Model file for the job. Use its own axes, mm. A direction names the side the tool comes from. Coordinates: 2 decimals unless noted, no trailing zeros. Order: outer loops, then holes, each group sorted by start corner. A loop starts at its lowest first (then second) coordinate and runs counter-clockwise, first axis right, second up. Notation, with made-up numbers: (-13, 10.5) -> (-4, 10.5) arc R32 ccw to (-4, 40.5) -> close; hole circle Ø10 at (55.5, -20). An arc over 180 degrees is marked (long way). Use CSV: the item, a comma, the result in double quotes. Start each with the question number.
(1) Cut at B-B on x = 20. Write the cut outline in (y, z), plus the area to 3 significant figures.
(2) Tool access for faces 4 (the flat face through (33, 19.05, -60)), 5 (the cylindrical face through (31.91, 9.392, -74.446)), 6 (the flat face through (33, 19.05, 59)): list every direction of +Z, -Z, +X, -X, +Y, -Y with a clear straight run to the whole face (end or side of a thin tool).
(3) Probe L1, parallel to Z at x = 38, y = 7; L2, parallel to Y at x = 50, z = -64.5; L3, parallel to Z at x = 21.5, y = 41. List the from-to ranges inside material, lowest first.
(4) Cut at A-A on x = 41. Write the cut outline in (y, z).
(5) Cut at C-C on y = 14.5. Give the number of separate pieces and of enclosed holes in the cut face, plus the area to 3 significant figures.
(6) Pull direction Z, two halves, no side cores. Call faces 1 (the cylindrical face through (48.74, 59.68, -1.02)), 2 (the cylindrical face through (31.715, 9.392, 74.433)), 3 (the cylindrical face through (42.34, 9.39, 52.64)): pulls with the +Z half, pulls with the -Z half, needs draft (parallel to the pull), parting line crosses it, or undercut.
(7) Pin check, flat tips, straight feed: pin 1 Ø1.3 at (x, y) = (42, 1.5) entering from -Z; pin 2 Ø24 at (x, z) = (29, -59) entering from +Y; pin 3 Ø12 at (x, y) = (36.5, 43) entering from +Z. Stop position of each tip, or through.
(8) Cut at D-D on z = 0. Write the cut outline in (x, y), plus the area to 3 significant figures.
```python
from build123d import *

# Parameters (mm, degrees)
SKETCH1_R               = 4.7625
SKETCH1_R_2             = 4.445
BOSS_EXTRUDE1_DEPTH     = 76.2
CUT_EXTRUDE6_DEPTH      = 61.487180317
CUT_EXTRUDE7_DEPTH      = 7.187819683
CUT_EXTRUDE7_DEPTH_BACK = 61.487180417
SKETCH10_R              = 9.525
CUT_EXTRUDE8_DEPTH      = 41.6400001


with BuildPart() as part:
    # Sketch1 → Boss-Extrude1 (new body)
    with BuildSketch(Plane(origin=(0, 0, 0), x_dir=(1, 0, 0), z_dir=(0, 1, 0))):
        with BuildLine():
            ThreePointArc((38.550556967, -72.995596152), (82.55, 0), (38.550556967, 72.995596152))
            ThreePointArc((38.550556967, 72.995596152), (31.812827991, 74.439846796), (25.312638114, 72.152843684))
            ThreePointArc((25.312638114, 72.152843684), (15.978447625, 56.116855626), (22.062819683, 38.588009636))
            ThreePointArc((22.062819683, 38.588009636), (44.45, 0), (22.062819683, -38.588009636))
            ThreePointArc((22.062819683, -38.588009636), (15.978447625, -56.116855626), (25.312638114, -72.152843684))
            ThreePointArc((25.312638114, -72.152843684), (31.812827991, -74.439846796), (38.550556967, -72.995596152))
        make_face()
        with Locations((38.1, 53.975)):
            Circle(SKETCH1_R, mode=Mode.SUBTRACT)
        with Locations((38.1, -53.975)):
            Circle(SKETCH1_R_2, mode=Mode.SUBTRACT)
    extrude(amount=BOSS_EXTRUDE1_DEPTH)

    # Sketch7 → Cut-Extrude6 (cut, through all)
    with BuildSketch(Plane.ZY.offset(-22.062819683)):
        with BuildLine():
            Line((-38.1, 2.54), (-38.1, 0))
            Line((-38.1, 0), (38.1, 0))
            Line((38.1, 0), (38.1, 2.54))
            ThreePointArc((38.1, 2.54), (0, 40.64), (-38.1, 2.54))
        make_face()
    extrude(amount=-CUT_EXTRUDE6_DEPTH, mode=Mode.SUBTRACT)

    # Sketch9 → Cut-Extrude7 (cut, two sides)
    with BuildSketch(Plane.ZY.offset(-22.062819683)) as cut_extrude7_sk:
        with BuildLine():
            Line((-74.465504436, 76.2), (-74.465504436, 19.05))
            Line((-74.465504436, 19.05), (-54.71327444, 19.05))
            ThreePointArc((-54.71327444, 19.05), (0, 59.69), (54.71327444, 19.05))
            Line((54.71327444, 19.05), (74.465504436, 19.05))
            Line((74.465504436, 19.05), (74.465504436, 76.2))
            Line((74.465504436, 76.2), (-74.465504436, 76.2))
        make_face()
    extrude(amount=CUT_EXTRUDE7_DEPTH, mode=Mode.SUBTRACT)
    extrude(cut_extrude7_sk.sketch, amount=-CUT_EXTRUDE7_DEPTH_BACK, mode=Mode.SUBTRACT)

    # Sketch10 → Cut-Extrude8 (cut, through all)
    with BuildSketch(Plane(origin=(0, 19.05, 0), x_dir=(1, 0, 0), z_dir=(0, 1, 0))):
        with Locations((38.1, 53.975)):
            Circle(SKETCH10_R)
        with Locations((38.1, -53.975)):
            Circle(SKETCH10_R)
    extrude(amount=CUT_EXTRUDE8_DEPTH, mode=Mode.SUBTRACT)


solid = part.part
```
Outcome:
1,outline,"(0, -66.87) -> (19.05, -66.87) -> (19.05, -54.71) arc R57.15 ccw to (42.27, -41.08) -> (0, -41.08) -> close; (0, 41.08) -> (42.27, 41.08) arc R57.15 ccw to (19.05, 54.71) -> (19.05, 66.87) -> (0, 66.87) -> close"
1,area,"1,360 mm2"
2,face 4,"-Z, +Y"
2,face 5,"-Z, +Y, -Y"
2,face 6,"+Z, +Y"
3,L1,"-73.27 to -58.74, -49.21 to -37.84, 37.84 to 49.53, 58.42 to 73.27"
3,L2,"0 to 19.05"
3,L3,"-42.27 to -39.2, 39.2 to 42.27"
4,outline,"(0, -71.65) -> (19.05, -71.65) -> (19.05, -57.75) -> (0, -57.75) -> close; (0, -50.2) -> (19.05, -50.2) -> (19.05, -44.9) -> (37.89, -44.9) arc R57.15 ccw to (57.05, -17.17) -> (36.55, -17.17) arc R38.1 cw to (2.54, -38.1) -> (0, -38.1) -> close; (0, 38.1) -> (2.54, 38.1) arc R38.1 cw to (36.55, 17.17) -> (57.05, 17.17) arc R57.15 ccw to (37.89, 44.9) -> (19.05, 44.9) -> (19.05, 50.61) -> (0, 50.61) -> close; (0, 57.34) -> (19.05, 57.34) -> (19.05, 71.65) -> (0, 71.65) -> close"
5,separate pieces,"2"
5,enclosed holes,"2"
5,area,"2,930 mm2"
6,face 1,"parting line crosses it"
6,face 2,"pulls with the +Z half"
6,face 3,"undercut"
7,pin 1,"z = -71.45"
7,pin 2,"y = 35.05"
7,pin 3,"z = 45.26"
8,outline,"(44.45, 40.64) -> (82.55, 40.64) -> (82.55, 59.69) -> (44.45, 59.69) -> close"
8,area,"726 mm2"
